from build123d import *

# Parameters (mm, degrees)
F4_DEPTH  = 12
F2_R      = 10
F5_DEPTH  = 6
F3_R      = 3.4
F6_DEPTH  = 18.001
F7_DEPTH  = 40
F9_R      = 14
F10_DEPTH = 50.001
F9_R_2    = 2.085835
F11_DEPTH = 20
F12_R     = 10
F13_DEPTH = 6
F14_DEPTH = 25


with BuildPart() as f4:
    # F1 (on face) → F4 (new body)
    with BuildSketch(Plane.XZ):
        with BuildLine():
            Line((51.534967, -13.733306), (29.534967, -13.733306))
            ThreePointArc((29.534967, -13.733306), (25.999433, -15.197772), (24.534967, -18.733306))
            Line((24.534967, -18.733306), (24.534967, -34.733306))
            ThreePointArc((24.534967, -34.733306), (25.999433, -38.26884), (29.534967, -39.733306))
            Line((29.534967, -39.733306), (51.534967, -39.733306))
            ThreePointArc((51.534967, -39.733306), (55.070501, -38.26884), (56.534967, -34.733306))
            Line((56.534967, -34.733306), (56.534967, -18.733306))
            ThreePointArc((56.534967, -18.733306), (55.070501, -15.197772), (51.534967, -13.733306))
        make_face()
    extrude(amount=F4_DEPTH)

    # F2 (on face) → F5 (join)
    with BuildSketch(Plane.XZ.offset(12)):
        with Locations((40.534967, -29.733306)):
            Circle(F2_R)
    extrude(amount=F5_DEPTH)

    # F3 (on face) → F6 (cut, through all)
    with BuildSketch(Plane.XZ):
        with Locations((40.534967, -29.733306)):
            Circle(F3_R)
    extrude(amount=F6_DEPTH, mode=Mode.SUBTRACT)

    # F0 (on Front) → F7 (join)
    with BuildSketch(Plane.XZ):
        with BuildLine():
            Line((63.719967, -4.733306), (17.719967, -4.733306))
            ThreePointArc((17.719967, -4.733306), (16.305754, -5.319092), (15.719967, -6.733306))
            Line((15.719967, -6.733306), (15.719967, -52.733306))
            ThreePointArc((15.719967, -52.733306), (16.305754, -54.147519), (17.719967, -54.733306))
            Line((17.719967, -54.733306), (63.719967, -54.733306))
            ThreePointArc((63.719967, -54.733306), (65.134181, -54.147519), (65.719967, -52.733306))
            Line((65.719967, -52.733306), (65.719967, -6.733306))
            ThreePointArc((65.719967, -6.733306), (65.134181, -5.319092), (63.719967, -4.733306))
        make_face()
    extrude(amount=-F7_DEPTH)

    # F9 (on face) → F10 (cut, through all)
    with BuildSketch(Plane(origin=(0, 0, -54.733306), x_dir=(1, 0, 0), z_dir=(0, 0, -1))):
        with Locations((40.719967, -20)):
            Circle(F9_R)
    extrude(amount=-F10_DEPTH, mode=Mode.SUBTRACT)

    # F9 (on face) → F11 (cut)
    with BuildSketch(Plane(origin=(0, 0, -54.733306), x_dir=(1, 0, 0), z_dir=(0, 0, -1))):
        with Locations((27.284938, -6.564971)):
            Circle(F9_R_2)
        with Locations((21.719967, -20)):
            Circle(F9_R_2)
        with Locations((27.284938, -33.435029)):
            Circle(F9_R_2)
        with Locations((54.154996, -6.564971)):
            Circle(F9_R_2)
        with Locations((59.719967, -20)):
            Circle(F9_R_2)
        with Locations((54.154996, -33.435029)):
            Circle(F9_R_2)
    extrude(amount=-F11_DEPTH, mode=Mode.SUBTRACT)

    # F12 (on face) → F13 (join)
    with BuildSketch(Plane.XZ):
        with Locations((40.534967, -29.733306)):
            Circle(F12_R)
    extrude(amount=F13_DEPTH)

    # F3 (on face) → F14 (cut)
    with BuildSketch(Plane.XZ):
        with Locations((40.534967, -29.733306)):
            Circle(F3_R)
    extrude(amount=F14_DEPTH, mode=Mode.SUBTRACT)


solid = f4.part
Geometry check sheet. Reference: the model listing, model coordinates, mm. A direction names the side the tool comes from. Round coordinates to 2 decimals unless told otherwise and drop trailing zeros. Loops run counter-clockwise (first coordinate to the right, second up) from the corner with the lowest first, then second, coordinate; pieces in that order, holes last. Notation, with made-up numbers: (2, -1) -> (40, -1) arc R19 ccw to (40, 21) -> close; hole circle Ø3 at (-2, 16.25). An arc over 180 degrees is marked (long way). Answer as a JSON object with one key per item and string values. Group by question number.
Item 1: Release check for a two-part mould opening along X. For faces 1 (the face through (50.073, -14.958, -26.73)), 2 (the face through (46, 6, -4.733)), 3 (the face through (54, 7, -34.733)), 4 (the face through (16.29, 19.72, -54.13)) record: pulls with the +X half, pulls with the -X half, needs draft (parallel to the pull), parting line crosses it, or undercut.
Item 2: Cross-section at D-D, the plane y = -2.5. Record the cut outline in (x, z).
Item 3: Cross-section at A-A, the plane y = 20. Record the cut outline in (x, z), plus the area to 3 significant figures.
Item 4: Set-up check for faces 5 (the face through (52.07, 6.47, -44.87)), 6 (the face through (40, 0, -40)), 7 (the face through (24.535, -6, -27)): record each of +Z, -Z, +X, -X, +Y, -Y from which the full face is reachable in a straight line by a thin tool's end or side.
Item 5: Cross-section at B-B, the plane x = 27.5. Record the cut outline in (y, z).
Item 6: Cross-section at C-C, the plane z = -32. Record the cut outline in (x, y).
Item 7: Depth check by flat-ended pin: pin 1 Ø1.5 at (x, z) = (40, -16.5) entering from -Y; pin 2 Ø9.5 at (x, y) = (42.5, -8) entering from -Z; pin 3 Ø25 at (x, y) = (40.72, 20) entering from +Z; pin 4 Ø1.5 at (x, z) = (27, -11) entering from -Y. Enter the tip coordinate at first touch or a pass-through.
Item 8: Thickness scan on line 1 along Y through (x, z) = (60, -37.5); line 2 along X through (y, z) = (5.5, -45.5); line 3 along X through (y, z) = (20, -27). Record the ranges inside material, lowest first.
Determined:
{
 "1": {"face 1": "parting line crosses it", "face 2": "needs draft", "face 3": "undercut", "face 4": "pulls with the -X half"},
 "2": {"outline": "(24.53, -34.73) arc R5 ccw to (29.53, -39.73) -> (51.53, -39.73) arc R5 ccw to (56.53, -34.73) -> (56.53, -18.73) arc R5 ccw to (51.53, -13.73) -> (29.53, -13.73) arc R5 ccw to (24.53, -18.73) -> close; hole circle Ø6.8 at (40.53, -29.73)"},
 "3": {"outline": "(15.72, -52.73) arc R2 ccw to (17.72, -54.73) -> (19.63, -54.73) -> (19.63, -34.73) -> (23.81, -34.73) -> (23.81, -54.73) -> (26.72, -54.73) -> (26.72, -4.73) -> (17.72, -4.73) arc R2 ccw to (15.72, -6.73) -> close; (54.72, -54.73) -> (57.63, -54.73) -> (57.63, -34.73) -> (61.81, -34.73) -> (61.81, -54.73) -> (63.72, -54.73) arc R2 ccw to (65.72, -52.73) -> (65.72, -6.73) arc R2 ccw to (63.72, -4.73) -> (54.72, -4.73) -> close", "area": "930 mm²"},
 "4": {"face 5": "-Z", "face 6": "-Y", "face 7": "+Z, -Z, -X, -Y"},
 "5": {"outline": "(-12, -39.3) -> (0, -39.3) -> (0, -54.73) -> (4.49, -54.73) -> (4.49, -34.73) -> (8.64, -34.73) -> (8.64, -54.73) -> (15.39, -54.73) -> (15.39, -4.73) -> (0, -4.73) -> (0, -14.17) -> (-12, -14.17) -> close; (24.61, -54.73) -> (31.36, -54.73) -> (31.36, -34.73) -> (35.51, -34.73) -> (35.51, -54.73) -> (40, -54.73) -> (40, -4.73) -> (24.61, -4.73) -> close"},
 "6": {"outline": "(15.72, 0) -> (24.53, 0) -> (24.53, -12) -> (30.8, -12) -> (30.8, -18) -> (38, -18) -> (38, 0) -> (43.07, 0) -> (43.07, -18) -> (50.27, -18) -> (50.27, -12) -> (56.53, -12) -> (56.53, 0) -> (65.72, 0) -> (65.72, 40) -> (15.72, 40) -> close; hole circle Ø28 at (40.72, 20)"},
 "7": {"pin 1": "stops at y = -12", "pin 2": "stops at z = -39.73", "pin 3": "passes through", "pin 4": "stops at y = 0"},
 "8": {"line 1": "y = 0 to 17.93, 22.07 to 40", "line 2": "x = 15.72 to 25.49, 29.08 to 52.36, 55.95 to 65.72", "line 3": "x = 15.72 to 26.72, 54.72 to 65.72"}
}
